from build123d import *

# Parameters (mm, degrees)
F0_R     = 1.55
F1_DEPTH = 3.175
F2_W     = 3.81
F2_H     = 1.905
F3_DEPTH = 12.7
F5_SIZE  = 3.556
F6_DEPTH = 4.445
F7_DEPTH = 4.445
F8_SIZE  = 0.9525
F9_DEPTH = 1.5875
F10_R    = 3.175


# Not quite as in the source:
# - a feature names something its author has since deleted; it is built from what else it names


with BuildPart() as f1:
    # F0 (on Top) → F1 (new body)
    with BuildSketch(Plane.XY):
        with BuildLine():
            ThreePointArc((10.25, 53.7461577598), (0, 43.4961577598), (-10.25, 53.7461577598))
            ThreePointArc((-10.25, 53.7461577598), (-10.7473318782, 55.3234929598), (-12.0594446059, 56.330312467))
            Line((-12.0594446059, 56.330312467), (-21.4563708137, 59.7505139002))
            ThreePointArc((-21.4563708137, 59.7505139002), (-23.5591264276, 59.6587056074), (-24.981080915, 58.1069145872))
            Line((-24.981080915, 58.1069145872), (-29.2563327066, 46.3607568274))
            ThreePointArc((-29.2563327066, 46.3607568274), (-29.3979964883, 45.0563146846), (-28.9191151455, 43.8347130349))
            Line((-28.9191151455, 43.8347130349), (-22.5348535878, 34.7870060575))
            ThreePointArc((-22.5348535878, 34.7870060575), (-19.9421017302, 29.5652521638), (-19.05, 23.803895516))
            Line((-19.05, 23.803895516), (-19.05, 0))
            Line((-19.05, 0), (19.05, 0))
            Line((19.05, 0), (19.05, 20.6116865479))
            ThreePointArc((19.05, 20.6116865479), (19.6246909156, 25.2555485437), (21.3140896836, 29.6192231062))
            Line((21.3140896836, 29.6192231062), (29.095340906, 44.1199008802))
            ThreePointArc((29.095340906, 44.1199008802), (29.4151082328, 45.2231386646), (29.2563327066, 46.3607568274))
            Line((29.2563327066, 46.3607568274), (24.981080915, 58.1069145872))
            ThreePointArc((24.981080915, 58.1069145872), (23.5591264276, 59.6587056074), (21.4563708137, 59.7505139002))
            Line((21.4563708137, 59.7505139002), (12.0594446059, 56.330312467))
            ThreePointArc((12.0594446059, 56.330312467), (10.7473318782, 55.3234929598), (10.25, 53.7461577598))
        make_face()
        with Locations((-17.2752517916, 42)):
            Circle(F0_R, mode=Mode.SUBTRACT)
        with Locations((-26.6721779994, 45.4202014333)):
            Circle(F0_R, mode=Mode.SUBTRACT)
        with Locations((-22.3969262079, 57.1663591931)):
            Circle(F0_R, mode=Mode.SUBTRACT)
        with Locations((-13, 53.7461577598)):
            Circle(F0_R, mode=Mode.SUBTRACT)
        with Locations((17.2752517916, 42)):
            Circle(F0_R, mode=Mode.SUBTRACT)
        with Locations((13, 53.7461577598)):
            Circle(F0_R, mode=Mode.SUBTRACT)
        with Locations((26.6721779994, 45.4202014333)):
            Circle(F0_R, mode=Mode.SUBTRACT)
        with Locations((22.3969262079, 57.1663591931)):
            Circle(F0_R, mode=Mode.SUBTRACT)
    extrude(amount=F1_DEPTH)

    # F2 (on face) → F3 (join)
    with BuildSketch(Plane.XZ):
        Polygon((14.2875, 7.9375), (14.2875, 3.175), (19.05, 3.175), (19.05, 10.4775), (10.7315, 10.4775), (10.7315, 7.9375), align=None)
        with Locations((0, 4.1275)):
            Rectangle(F2_W, F2_H)
        Polygon((-19.05, 3.175), (-14.2875, 3.175), (-14.2875, 7.9375), (-10.7315, 7.9375), (-10.7315, 10.4775), (-19.05, 10.4775), align=None)
    extrude(amount=-F3_DEPTH)

    # F4: F1 across face


with BuildPart() as f1_1:
    add(f1.part)
    add(f1.part.mirror(Plane(origin=(0, 0, 3.9988214553), x_dir=(1, 0, 0), z_dir=(0, -1, 0))))

    # F5
    f5_edges = [f1_1.edges().sort_by_distance(p)[0] for p in [
        (10.7315, -12.7, 9.2075),
        (-10.7315, -12.7, 9.2075),
        (-10.7315, 12.7, 9.2075),
        (10.7315, 12.7, 9.2075),
    ]]
    chamfer(f5_edges, length=F5_SIZE)

    # F6 (add): a face of the model
    f6_faces = [f1_1.faces().sort_by_distance(p)[0] for p in [
        (0, -12.7, 4.1275),
    ]]
    extrude(f6_faces, amount=F6_DEPTH)

    # F7 (add): a face of the model
    f7_faces = [f1_1.faces().sort_by_distance(p)[0] for p in [
        (0, 12.7, 4.1275),
    ]]
    extrude(f7_faces, amount=F7_DEPTH)

    # F8
    f8_edges = [f1_1.edges().sort_by_distance(p)[0] for p in [
        (0, 17.145, 5.08),
        (0, -17.145, 5.08),
    ]]
    chamfer(f8_edges, length=F8_SIZE)

    # F9 (cut): a face of the model
    f9_faces = [f1_1.faces().sort_by_distance(p)[0] for p in [
        (0.1994717604, 0, 0),
    ]]
    extrude(f9_faces, amount=-F9_DEPTH, mode=Mode.SUBTRACT)

    # F10
    f10_edges = [f1_1.edges().sort_by_distance(p)[0] for p in [
        (-19.05, 0, 10.4775),
        (19.05, 0, 10.4775),
    ]]
    fillet(f10_edges, radius=F10_R)


solid = f1_1.part
Here's how the part is built. I have some questions about the finished solid (model axes, mm). A direction names the side the tool comes from. Give positions to 0.01 mm unless a question says otherwise; leave off trailing zeros. Loops run counter-clockwise (first coordinate to the right, second up) from the corner with the lowest first, then second, coordinate; pieces in that order, holes last. Notation, with made-up numbers: (62.25, -9) -> (67.25, -9) arc R20 cw to (67.25, 14) -> close; hole circle Ø5 at (-9.5, 18.5). An arc over 180 degrees is marked (long way). Answer as a JSON object with one key per item and string values. Group by question number.
Item 1: Will these pins go through, and if not, where does the flat tip stop? pin 1 (1.5 mm diameter, centred on x = -15, y = -16.5, fed in from +Z) (3 decimals); pin 2 (5 mm diameter, centred on y = -1.5, z = 9.5, fed in from +X); pin 3 (1.9 mm diameter, centred on x = 22.4, y = 57.17, fed in from -Z); pin 4 (12 mm diameter, centred on x = -2, y = -14.5, fed in from +Z).
Item 2: Imagine slicing it at C-C on x = 0. Write out the boundary of the cut face in (y, z) (1 decimal), then the cut area to 3 significant figures.
Item 3: Imagine slicing it at D-D on y = 42. Write out the boundary of the cut face in (x, z) (1 decimal).
Item 4: On a 3-axis mill with a long thin cutter (end or side, diameter ignored), from which of +Z, -Z, +X, -X, +Y, -Y can I reach the whole of each face in a straight line? I mean faces 4 (the flat face through (-12.485, 10.897, 9.19)), 5 (the flat face through (-16.692, 58.016, 2.37)), 6 (the flat face through (-25.77, 39.37, 2.37)), 7 (the flat face through (0, 0, 5.08)), 8 (the flat face through (17, -12.7, 7)). Say none if no direction works.
Item 5: Imagine slicing it at B-B on x = -17.5. Write out the boundary of the cut face in (y, z) (1 decimal).
Item 6: Thinking about a two-plate mould opening in X: for faces 1 (the flat face through (-27.089, -52.316, 2.37)), 2 (the flat face through (13, 0, 10.478)), 3 (the cylindrical face through (0.2, -43.5, 2.4)), which applies, pulls with the +X half, pulls with the -X half, needs draft (parallel to the pull), parting line crosses it, or undercut?
Item 7: I need wall thicknesses on L1, parallel to X at y = -5.5, z = 5.75; L2, parallel to Y at x = 19, z = 4.25; L3, parallel to X at y = -42, z = 2.3. Which ranges of each line are inside material? Lowest first, please.
Answer list:
{
 "1": {"pin 1": "stops at z = 3.175", "pin 2": "stops at x = 19.05", "pin 3": "passes through", "pin 4": "stops at z = 5.08"},
 "2": {"outline": "(-43.5, 1.6) -> (43.5, 1.6) -> (43.5, 3.2) -> (17.1, 3.2) -> (17.1, 4.1) -> (16.2, 5.1) -> (-16.2, 5.1) -> (-17.1, 4.1) -> (-17.1, 3.2) -> (-43.5, 3.2) -> close", "area": "203 mm2"},
 "3": {"outline": "(-27.6, 1.6) -> (-18.8, 1.6) -> (-18.8, 3.2) -> (-27.6, 3.2) -> close; (-15.7, 1.6) -> (15.7, 1.6) -> (15.7, 3.2) -> (-15.7, 3.2) -> close; (18.8, 1.6) -> (28, 1.6) -> (28, 3.2) -> (18.8, 3.2) -> close"},
 "4": {"face 4": "+Z, +Y", "face 5": "+Z, -Z, +Y", "face 6": "+Z, -Z, -X", "face 7": "+Z, +Y, -Y", "face 8": "+Z, +X, -Y"},
 "5": {"outline": "(-58.3, 1.6) -> (-43.5, 1.6) -> (-43.5, 3.2) -> (-58.3, 3.2) -> close; (-40.5, 1.6) -> (40.5, 1.6) -> (40.5, 3.2) -> (12.7, 3.2) -> (12.7, 10) -> (-12.7, 10) -> (-12.7, 3.2) -> (-40.5, 3.2) -> close; (43.5, 1.6) -> (58.3, 1.6) -> (58.3, 3.2) -> (43.5, 3.2) -> close"},
 "6": {"face 1": "pulls with the -X half", "face 2": "needs draft", "face 3": "undercut"},
 "7": {"L1": "x = -19.05 to -14.29, 14.29 to 19.05", "L2": "y = -12.7 to 12.7", "L3": "x = -27.62 to -18.83, -15.73 to 15.73, 18.83 to 27.96"}
}
